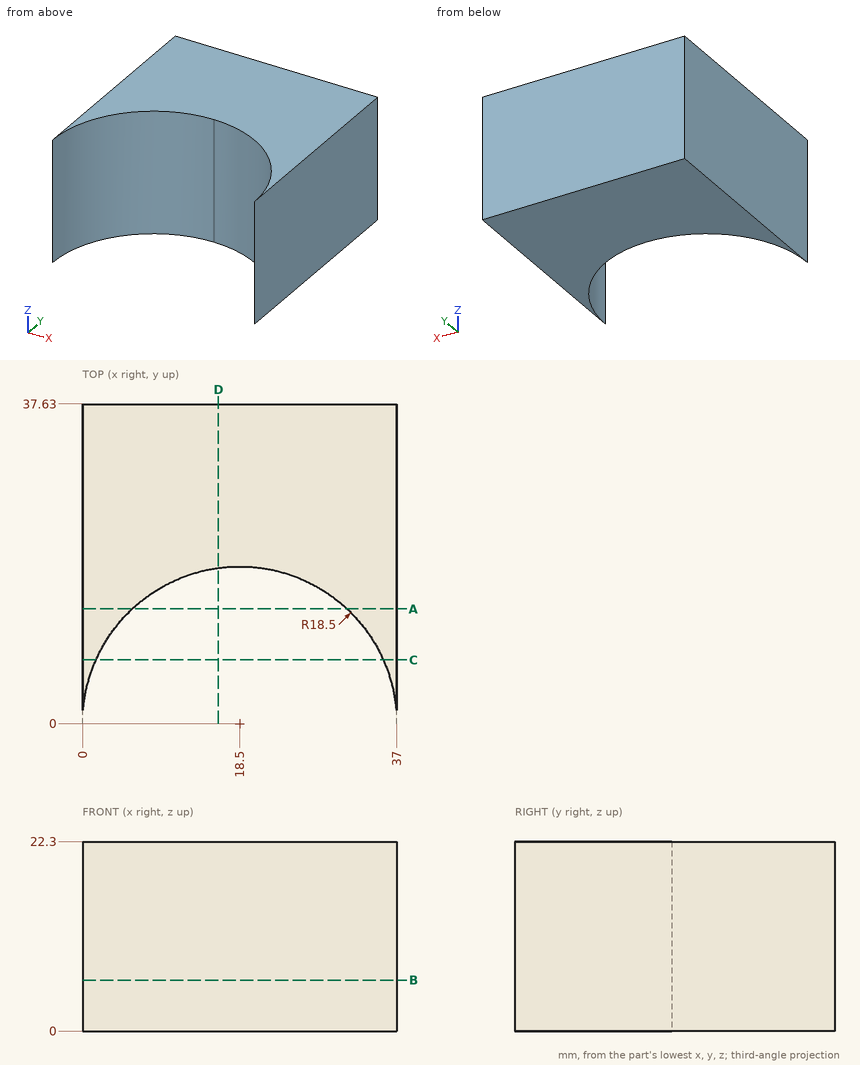
For this review, use the dimensioned drawing (mm, ordinates from the lowest corner) and the shaded views. Give positions to 0.01 mm unless a question says otherwise; leave off trailing zeros. Order: outer loops, then holes, each group sorted by start corner. A loop starts at its lowest first (then second) coordinate and runs counter-clockwise, first axis right, second up. Notation, with made-up numbers: M 42,2.25 L 76,2.25 A24 ccw 76,25.25 Z; hole C 61.25,-5.5 d11. An arc over 180 degrees is marked long. Use one line per item in the form item = value. Start each with the question number.
Item 1: We need section B-B on z = 6. Give the boundary of the cut face in (x, y).
Item 2: We need section D-D on x = 16. Give the boundary of the cut face in (y, z), plus the area to 3 significant figures.
Item 3: To check wall thickness, follow line 1 along X through (y, z) = (7, 18); line 2 along X through (y, z) = (8, 12.75); line 3 along Y through (x, z) = (18, 16.75). State the ranges of each line that lie inside material, in increasing order. Write a range as from..to.
Item 4: We need section C-C on y = 7.5. Give the boundary of the cut face in (x, z), plus the area to 3 significant figures.
Item 5: Insertion check: pin 1 Ø6 at (x, z) = (30, 17.5) entering from -Y; pin 2 Ø10 at (x, z) = (26.5, 20) entering from -Y; pin 3 Ø1 at (x, z) = (24, 4.5) entering from -Y. Each pin has a flat end and moves straight along its axis. Give the tip position at first contact, or say it passes through.
Item 6: We need section A-A on y = 13.5. Give the boundary of the cut face in (x, z), plus the area to 3 significant figures.
Completed:
q1.outline = M 0,0 A18.5 cw 37,0 L 37,37.63 L 0,37.63 Z
q2.outline = M 18.33,0 L 37.63,0 L 37.63,22.3 L 18.33,22.3 Z
q2.area = 430 mm²
q3.line_1 = 0..1.38, 35.62..37
q3.line_2 = 0..1.82, 35.18..37
q3.line_3 = 18.49..37.63
q4.outline = M 0,0 L 1.59,0 L 1.59,22.3 L 0,22.3 Z; M 35.41,0 L 37,0 L 37,22.3 L 35.41,22.3 Z
q4.area = 70.8 mm²
q5.pin_1 = 11.49
q5.pin_2 = 13.16
q5.pin_3 = 17.5
q6.outline = M 0,0 L 5.85,0 L 5.85,22.3 L 0,22.3 Z; M 31.15,0 L 37,0 L 37,22.3 L 31.15,22.3 Z
q6.area = 261 mm²
